The listing builds one solid part. Answer for the finished solid, in the listing's coordinates (mm). A direction names the side the tool comes from. Coordinates: 2 decimals unless noted, no trailing zeros. Order: outer loops, then holes, each group sorted by start corner. A loop starts at its lowest first (then second) coordinate and runs counter-clockwise, first axis right, second up. Notation, with made-up numbers: (-21.5, 13) -> (-14.5, 13) arc R18 cw to (-14.5, 23) -> close; hole circle Ø7 at (6, -9.75). An arc over 180 degrees is marked (long way). Answer in a Markdown table with one row per item.
```python
from build123d import *
from build123d.topology import SkipClean

# Parameters (mm, degrees)
SKETCH_1_R          = 46.9
SKETCH_1_R_2        = 40.9
SKETCH_1_R_3        = 1.6
EXTRUDE_1_DEPTH     = 20.5
SKETCH_2_R          = 3
EXTRUDE_2_DEPTH     = 20.5
SKETCH_3_R          = 1.6
CUT_EXTRUDE_1_DEPTH = 25
CUT_EXTRUDE_START   = -25
CUT_EXTRUDE_2_DEPTH = 25
CUT_EXTRUDE_3_DEPTH = 67.780389508


with BuildPart() as part:
    # 草图1 → 凸台-拉伸1 (new body)
    with BuildSketch(Plane(origin=(0, 0, 0), x_dir=(1, 0, 0), z_dir=(0, 1, 0))):
        with Locations(Location((0, 0, 0), (0, 0, 270))):
            Circle(SKETCH_1_R)
        with Locations(Location((0, 0, 0), (0, 0, 270))):
            Circle(SKETCH_1_R_2, mode=Mode.SUBTRACT)
        with Locations(Location((12.835117837, 41.981778787, 0), (0, 0, 270))):
            Circle(SKETCH_1_R_3, mode=Mode.SUBTRACT)
        with Locations(Location((-17.153096541, 40.410163067, 0), (0, 0, 270))):
            Circle(SKETCH_1_R_3, mode=Mode.SUBTRACT)
    extrude(amount=EXTRUDE_1_DEPTH)

    # 草图2 → 凸台-拉伸2 (add)
    with BuildSketch(Plane(origin=(0, 20.5, 0), x_dir=(1, 0, 0), z_dir=(0, 1, 0))):
        with Locations((31.749094475, 31.749094475)):
            Circle(SKETCH_2_R)
        with Locations((31.749094475, -31.749094475)):
            Circle(SKETCH_2_R)
        with Locations((-31.749094475, -31.749094475)):
            Circle(SKETCH_2_R)
        with Locations((-31.749094475, 31.749094475)):
            Circle(SKETCH_2_R)
    extrude(amount=-EXTRUDE_2_DEPTH)

    # 草图3 → 切除-拉伸1 (cut)
    with BuildSketch(Plane(origin=(0, 20.5, 0), x_dir=(1, 0, 0), z_dir=(0, 1, 0))):
        with Locations(Location((-31.749094475, 31.749094475, 0), (0, 0, 270))):
            Circle(SKETCH_3_R)
        with Locations(Location((-31.749094475, -31.749094475, 0), (0, 0, 270))):
            Circle(SKETCH_3_R)
        with Locations(Location((31.749094475, -31.749094475, 0), (0, 0, 270))):
            Circle(SKETCH_3_R)
        with Locations(Location((31.749094475, 31.749094475, 0), (0, 0, 270))):
            Circle(SKETCH_3_R)
    extrude(amount=-CUT_EXTRUDE_1_DEPTH, mode=Mode.SUBTRACT)

    # 草图4 → 切除-拉伸2 (cut)
    with SkipClean():  # the faces are left unmerged after this step: merging them gives an invalid solid
        with BuildSketch(Plane(origin=(0, 20.5, 0), x_dir=(1, 0, 0), z_dir=(0, 1, 0)).offset(CUT_EXTRUDE_START)):
            with BuildLine():
                ThreePointArc((-20.139957039, 40.129691383), (-19.729499495, 41.947091113), (-18.325289788, 43.171677686))
                ThreePointArc((-18.325289788, 43.171677686), (-25.271051327, 39.509289602), (-31.508446668, 34.739427004))
                ThreePointArc((-31.508446668, 34.739427004), (-30.445394472, 34.451013479), (-29.558090066, 33.798362559))
                ThreePointArc((-29.558090066, 33.798362559), (-25.049858336, 37.262777638), (-20.139957039, 40.129691383))
            make_face()
            with BuildLine():
                ThreePointArc((10.366766227, 43.686841932), (11.849397191, 44.815213947), (13.71223353, 44.850692878))
                ThreePointArc((13.71223353, 44.850692878), (-2.454555971, 46.8357252), (-18.325289788, 43.171677686))
                ThreePointArc((-18.325289788, 43.171677686), (-16.468950031, 43.331112151), (-14.876494449, 42.363898698))
                ThreePointArc((-14.876494449, 42.363898698), (-2.349884435, 44.83846611), (10.366766227, 43.686841932))
            make_face()
            with BuildLine():
                ThreePointArc((29.558090066, 33.798362559), (30.445394472, 34.451013479), (31.508446668, 34.739427004))
                ThreePointArc((31.508446668, 34.739427004), (23.168662106, 40.777727943), (13.71223353, 44.850692878))
                ThreePointArc((13.71223353, 44.850692878), (15.236754486, 43.77959452), (15.834933275, 42.015055494))
                ThreePointArc((15.834933275, 42.015055494), (23.065345276, 38.522718586), (29.558090066, 33.798362559))
            make_face()
            with BuildLine():
                ThreePointArc((33.798362559, -29.558090066), (44.9, 0), (33.798362559, 29.558090066))
                ThreePointArc((33.798362559, 29.558090066), (34.451013479, 30.445394472), (34.739427004, 31.508446668))
                ThreePointArc((34.739427004, 31.508446668), (46.9, 0), (34.739427004, -31.508446668))
                ThreePointArc((34.739427004, -31.508446668), (34.451013479, -30.445394472), (33.798362559, -29.558090066))
            make_face()
            with BuildLine():
                ThreePointArc((-33.798362559, -29.558090066), (-34.451013479, -30.445394472), (-34.739427004, -31.508446668))
                ThreePointArc((-34.739427004, -31.508446668), (-46.9, 0), (-34.739427004, 31.508446668))
                ThreePointArc((-34.739427004, 31.508446668), (-34.451013479, 30.445394472), (-33.798362559, 29.558090066))
                ThreePointArc((-33.798362559, 29.558090066), (-44.9, 0), (-33.798362559, -29.558090066))
            make_face()
            with BuildLine():
                ThreePointArc((-31.508446668, -34.739427004), (-30.445394472, -34.451013479), (-29.558090066, -33.798362559))
                ThreePointArc((-29.558090066, -33.798362559), (0, -44.9), (29.558090066, -33.798362559))
                ThreePointArc((29.558090066, -33.798362559), (30.445394472, -34.451013479), (31.508446668, -34.739427004))
                ThreePointArc((31.508446668, -34.739427004), (0, -46.9), (-31.508446668, -34.739427004))
            make_face()
        extrude(amount=CUT_EXTRUDE_2_DEPTH, mode=Mode.SUBTRACT)

    # 草图5 → 切除-拉伸3 (cut, through all)
    with SkipClean():  # the faces are left unmerged after this step: merging them gives an invalid solid
        with BuildSketch(Plane.XY):
            with BuildLine():
                Line((-3.5, 3.5), (-3.5, 0))
                Line((-3.5, 0), (3.5, 0))
                Line((3.5, 0), (3.5, 3.5))
                ThreePointArc((3.5, 3.5), (0, 7), (-3.5, 3.5))
            make_face()
        extrude(amount=CUT_EXTRUDE_3_DEPTH, mode=Mode.SUBTRACT)


solid = part.part
```
(1) A cutting plane is placed at A-A, the plane x = 0. Determine the outline of the cut face in (y, z).
Check values:
| item | result |
|---|---|
| outline | (0, -44.9) -> (20.5, -44.9) -> (20.5, -40.9) -> (0, -40.9) -> close; (7, 40.9) -> (20.5, 40.9) -> (20.5, 44.9) -> (7, 44.9) -> close |
(2) A cutting plane is placed at B-B, the plane z = 0. Determine the outline of the cut face in (x, y).
Check values:
| item | result |
|---|---|
| outline | (-44.9, 0) -> (-40.9, 0) -> (-40.9, 20.5) -> (-44.9, 20.5) -> close; (40.9, 0) -> (44.9, 0) -> (44.9, 20.5) -> (40.9, 20.5) -> close |
(3) Find the intervals of material crossed by line 1 along Z through (x, y) = (31, 6.25); line 2 along X through (y, z) = (9, 0.5); line 3 along Z through (x, y) = (-17.5, 16.25), in increasing order. Write a range as from..to.
Check values:
| item | result |
|---|---|
| line 1 | -34.65..-33.16, -30.34..-26.68, 26.68..30.34, 33.16..34.65 |
| line 2 | -44.9..-40.9, 40.9..44.9 |
| line 3 | -43.39..-41.97, -38.85..-36.97, 36.97..41.35 |
(4) A cutting plane is placed at C-C, the plane y = 16.25. Determine the outline of the cut face in (x, z), then the cut area to 3 significant figures.
Check values:
| item | result |
|---|---|
| outline | (-33.8, -29.56) arc R3 ccw (long way) to (-29.56, -33.8) arc R44.9 ccw to (-20.14, -40.13) arc R3 ccw to (-14.88, -42.36) arc R44.9 ccw to (10.37, -43.69) arc R3 ccw to (15.83, -42.02) arc R44.9 ccw to (29.56, -33.8) arc R3 ccw (long way) to (33.8, -29.56) arc R44.9 ccw to (33.8, 29.56) arc R3 ccw (long way) to (29.56, 33.8) arc R44.9 ccw to (-29.56, 33.8) arc R3 ccw (long way) to (-33.8, 29.56) arc R44.9 ccw to start; hole circle Ø81.8 at (0, 0); hole circle Ø3.2 at (-31.75, -31.75); hole circle Ø3.2 at (-31.75, 31.75); hole circle Ø3.2 at (-17.15, -40.41); hole circle Ø3.2 at (12.84, -41.98); hole circle Ø3.2 at (31.75, -31.75); hole circle Ø3.2 at (31.75, 31.75) |
| area | 1,100 mm² |
(5) For a pull along X with two mould halves and no side action, classify faces 3 (the flat face through (-40, 20.5, 10)), 4 (the cylindrical face through (-44.898, 10.106, -0.452)), 5 (the cylindrical face through (40.552, 10.106, -5.324)) as released by +X, released by -X, zero draft, split by the parting line, or undercut.
Check values:
| item | result |
|---|---|
| face 3 | zero draft |
| face 4 | released by -X |
| face 5 | undercut |
(6) Flat-ended cylindrical pins translate along their axes: pin 1 (5 mm diameter, centred on x = -17, y = 2.5, fed in from -Z); pin 2 (3 mm diameter, centred on y = 1, z = 43, fed in from -X); pin 3 (12 mm diameter, centred on x = 18.5, y = 13, fed in from +Z). Find the tip coordinate at first contact, or state that the pin passes through.
Check values:
| item | result |
|---|---|
| pin 1 | z = -43.41 |
| pin 2 | x = -17.14 |
| pin 3 | z = 43.12 |
(7) Which of the six approach directions +Z, -Z, +X, -X, +Y, -Y give full straight-line access (tool end or side, diameter ignored) to faces 1 (the cylindrical face through (-31.268, 10.394, 33.275)), 2 (the flat face through (-3.5, 2, 43))?
Check values:
| item | result |
|---|---|
| face 1 | +Y, -Y |
| face 2 | +Z, -Y |
